Here's how the part is built. I have some questions about the finished solid (model axes, mm). A direction names the side the tool comes from. Give positions to 0.01 mm unless a question says otherwise; leave off trailing zeros. Write each loop counter-clockwise with the first axis right and the second up, starting at its lowest first coordinate (ties: lowest second). Pieces come first, ordered by that corner, then holes. Notation, with made-up numbers: (76, 8) -> (134, 8) arc R20 cw to (134, 45) -> close; hole circle Ø7 at (73, 89). An arc over 180 degrees is marked (long way). Answer as CSV lines item,"result". Start each with the question number.
from build123d import *

# Parameters (mm, degrees)
SKETCH2_W             = 25.7
SKETCH2_H             = 17.88
BOSS_EXTRUDE1_DEPTH   = 0.9
SKETCH3_W             = 17.6
SKETCH3_H             = 15.8
BOSS_EXTRUDE2_DEPTH   = 2.15
F_1_5MM_DOWEL_HOLE1_D = 0.6


with BuildPart() as part:
    # Sketch2 → Boss-Extrude1 (new body)
    with BuildSketch(Plane(origin=(0, 0, 0), x_dir=(1, 0, 0), z_dir=(0, 1, 0))):
        Rectangle(SKETCH2_W, SKETCH2_H)
    extrude(amount=BOSS_EXTRUDE1_DEPTH)

    # Sketch3 → Boss-Extrude2 (add)
    with BuildSketch(Plane(origin=(0, 0.9, 0), x_dir=(1, 0, 0), z_dir=(0, 1, 0))):
        with Locations((3.05, 0)):
            Rectangle(SKETCH3_W, SKETCH3_H)
    extrude(amount=BOSS_EXTRUDE2_DEPTH)

    # Ø1.5mm Dowel Hole1 (through all)
    with Locations(Plane(origin=(0, 3.05, 0), x_dir=(1, 0, 0), z_dir=(0, 1, 0))):
        with Locations((11.35, 8.94), (10.1, 8.94), (8.85, 8.94), (7.6, 8.94), (6.35, 8.94), (5.1, 8.94), (3.85, 8.94), (2.6, 8.94), (1.35, 8.94), (0.1, 8.94), (-1.15, 8.94), (-2.4, 8.94), (-3.65, 8.94), (-4.9, 8.94), (11.35, -8.94), (10.1, -8.94), (8.85, -8.94), (7.6, -8.94), (6.35, -8.94), (5.1, -8.94), (3.85, -8.94), (2.6, -8.94), (1.35, -8.94), (0.1, -8.94), (-1.15, -8.94), (-2.4, -8.94), (-3.65, -8.94), (-4.9, -8.94), (12.85, 5.64), (12.85, 4.39), (12.85, 3.14), (12.85, 1.89), (12.85, 0.64), (12.85, -0.61), (12.85, -1.86), (12.85, -3.11), (12.85, -4.36), (12.85, -5.61)):
            Hole(F_1_5MM_DOWEL_HOLE1_D / 2)


solid = part.part
Item 1: If we section it at A-A (z = 6.75): Please give me the cut outline in (x, y).
Item 2: If we section it at D-D (x = -8.25): Please give me the cut outline in (y, z), and give its area (3 significant figures).
Item 3: I'm going to push flat-ended pins straight in: pin 1 (1.7 mm diameter, centred on x = 3.5, y = 2.5, fed in from -Z); pin 2 (1.1 mm diameter, centred on x = 2.5, y = 2.5, fed in from +Z); pin 3 (3 mm diameter, centred on x = 5, z = 7, fed in from -Y); pin 4 (1.1 mm diameter, centred on y = 2, z = 4, fed in from +X). Where does each tip first touch, or does it pass through?
Item 4: If we section it at B-B (x = -3.65): Please give me the cut outline in (y, z), and give its area (3 significant figures).
Item 5: We'd pull the mould along X, two halves only. Please class faces 1 (the face through (-6, 0.9, -2)), 2 (the face through (-5.75, 2, 0)), 3 (the face through (12.85, 0.4, 7.4)): released by +X, released by -X, zero draft, split by the parting line, or undercut.
Item 6: If we section it at C-C (y = 2.6): Please give me the cut outline in (x, z), and give its area (3 significant figures).
Item 7: For faces 4 (the face through (11.85, 2, 0)), 5 (the face through (-12.85, 0.4, 0.1)), 6 (the face through (12.85, 0.4, -7.4)), 7 (the face through (3, 2, -7.9)), 8 (the face through (3, 2, 7.9)), which set-ups out of +Z, -Z, +X, -X, +Y, -Y let a thin tool reach every point of the face, with its end or its side?
Item 8: If I drill on line 1 (X direction, y = 2.95, z = 4.25); line 2 (Z direction, x = -3, y = 2.2); line 3 (Y direction, x = -11, z = -7.25), over which ranges is the centre line in solid material (lowest first)? Write a range as [from, to].
Final values:
1,outline,"(-12.85, 0) -> (12.85, 0) -> (12.85, 0.9) -> (11.85, 0.9) -> (11.85, 3.05) -> (-5.75, 3.05) -> (-5.75, 0.9) -> (-12.85, 0.9) -> close"
2,outline,"(0, -8.94) -> (0.9, -8.94) -> (0.9, 8.94) -> (0, 8.94) -> close"
2,area,"16.1 mm2"
3,pin 1,"z = -7.9"
3,pin 2,"z = 7.9"
3,pin 3,"y = 0"
3,pin 4,"x = 11.85"
4,outline,"(0, -8.64) -> (0.9, -8.64) -> (0.9, -7.9) -> (3.05, -7.9) -> (3.05, 7.9) -> (0.9, 7.9) -> (0.9, 8.64) -> (0, 8.64) -> close"
4,area,"49.5 mm2"
5,face 1,"zero draft"
5,face 2,"released by -X"
5,face 3,"released by +X"
6,outline,"(-5.75, -7.9) -> (11.85, -7.9) -> (11.85, 7.9) -> (-5.75, 7.9) -> close"
6,area,"278 mm2"
7,face 4,"+Z, -Z, +X, +Y"
7,face 5,"+Z, -Z, -X, +Y, -Y"
7,face 6,"+Z, -Z, +X, +Y, -Y"
7,face 7,"-Z, +X, -X, +Y"
7,face 8,"+Z, +X, -X, +Y"
8,line 1,"[-5.75, 11.85]"
8,line 2,"[-7.9, 7.9]"
8,line 3,"[0, 0.9]"
